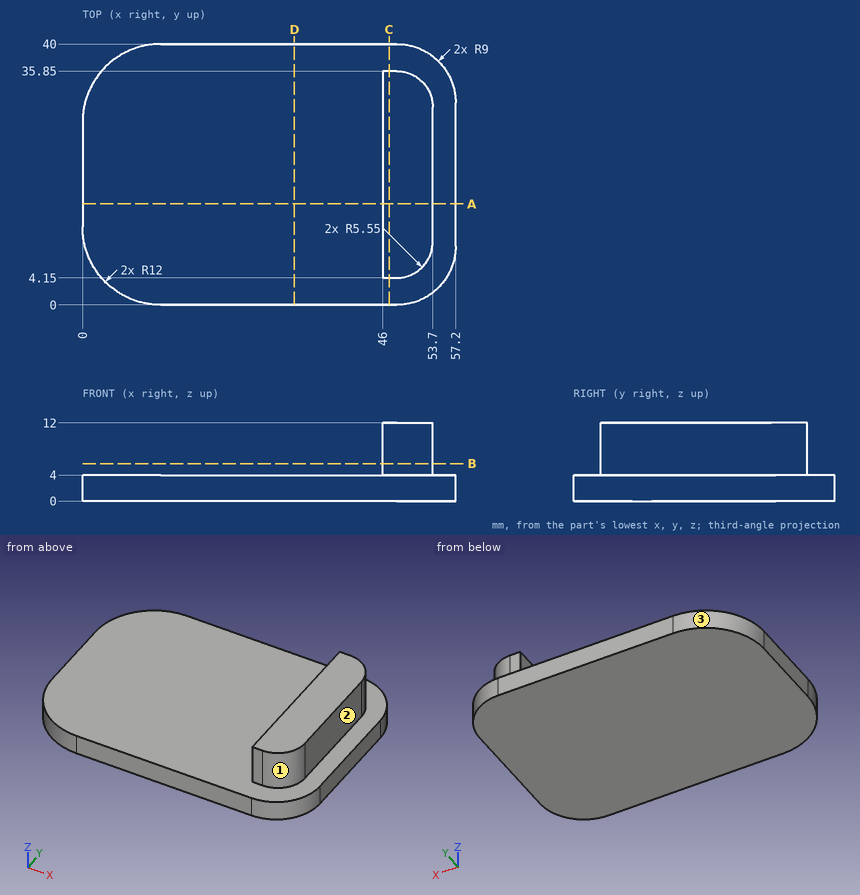
Geometry check sheet. Reference: drawing and pictorial views, mm from the part's lowest x, y, z. A direction names the side the tool comes from. Round coordinates to 2 decimals unless told otherwise and drop trailing zeros. Order: outer loops, then holes, each group sorted by start corner. A loop starts at its lowest first (then second) coordinate and runs counter-clockwise, first axis right, second up. Notation, with made-up numbers: M 1.25,83.25 L 56.25,83.25 A11 ccw 56.25,99.25 Z; hole C 43.5,79 d6. An arc over 180 degrees is marked long. Write item = value, one per line.
Q1. Section check B-B (z = 5.75). Enter the section's corners in (x, y), plus the area to 3 significant figures.
Answer block:
outline = M 46,4.15 L 48.15,4.15 A5.55 ccw 53.7,9.7 L 53.7,30.3 A5.55 ccw 48.15,35.85 L 46,35.85 Z
area = 231 mm^2
Q2. Depth check by flat-ended pin: pin 1 Ø3 at (y, z) = (14, 7.5) entering from -X; pin 2 Ø1.1 at (x, z) = (47, 7.5) entering from +Y; pin 3 Ø3 at (y, z) = (10.5, 7) entering from +X. Enter the tip coordinate at first touch or a pass-through.
Answer block:
pin_1 = 46
pin_2 = 35.85
pin_3 = 53.7
Q3. Set-up check for the marked faces 1, 2 and 3: record each of +Z, -Z, +X, -X, +Y, -Y from which the full face is reachable in a straight line by a thin tool's end or side.
Answer block:
face_1 = +Z, +X, -Y
face_2 = +Z, +X, +Y, -Y
face_3 = +Z, -Z, -X, +Y
Q4. Section check D-D (x = 32.5). Enter the section's corners in (y, z).
Answer block:
outline = M 0,0 L 40,0 L 40,4 L 0,4 Z
Q5. Section check C-C (x = 47). Enter the section's corners in (y, z), plus the area to 3 significant figures.
Answer block:
outline = M 0,0 L 40,0 L 40,4 L 35.85,4 L 35.85,12 L 4.15,12 L 4.15,4 L 0,4 Z
area = 414 mm^2
Q6. Section check A-A (y = 15.5). Enter the section's corners in (x, z).
Answer block:
outline = M 0,0 L 57.2,0 L 57.2,4 L 53.7,4 L 53.7,12 L 46,12 L 46,4 L 0,4 Z
Q7. Scan lines: line 1 (Z direction, x = 7.5, y = 17.5); line 2 (X direction, y = 19, z = 4.5); line 3 (Y direction, x = 48, z = 9.25). Record each from-to range of solid material in increasing order.
Answer block:
line_1 = 0 to 4
line_2 = 46 to 53.7
line_3 = 4.15 to 35.85
